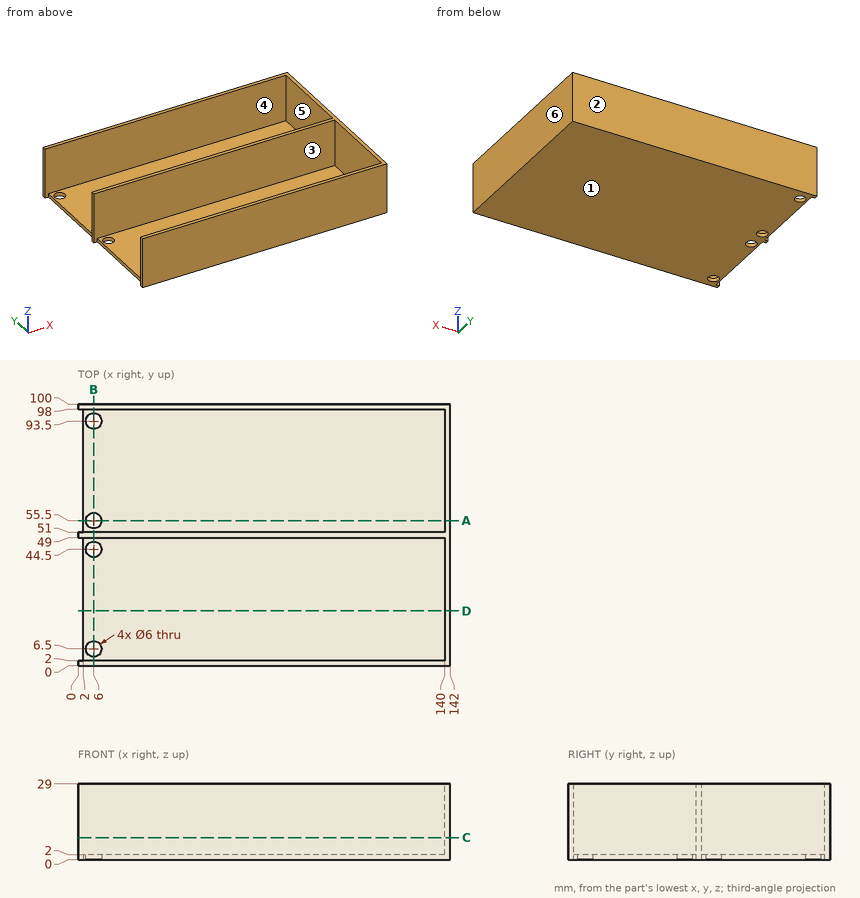
Input: dimensioned drawing with shaded views. Units: mm. Origin: part minimum x, y, z. A direction names the side the tool comes from. Coordinates: 2 decimals unless noted, no trailing zeros. Write each loop counter-clockwise with the first axis right and the second up, starting at its lowest first coordinate (ties: lowest second). Pieces come first, ordered by that corner, then holes. Notation, with made-up numbers: (27, 41) -> (80, 41) arc R37 cw to (80, 79) -> close; hole circle Ø5 at (64.5, 28). An arc over 180 degrees is marked (long way). Return JSON: item names as keys, results as strings. Group by question number.
1) Section query B-B, the plane x = 6. Return loops of the section in (y, z).
2) Section query D-D, the plane y = 21. Return loops of the section in (x, z), plus the area to 3 significant figures.
3) Section query C-C, the plane z = 8.5. Return loops of the section in (x, y), plus the area to 3 significant figures.
4) Contact query for flat-ended pins moving along their axis: P1, Ø14.5, axis at x = 97.5, z = 20, coming from the -Y side; P2, Ø8, axis at x = 6, y = 6.5, coming from the +Z side; P3, Ø0.6, axis at y = 72, z = 1, coming from the -X side; P4, Ø1, axis at y = 81.5, z = 16.5, coming from the -X side. Output: stop coordinate, or through.
5) Set-up query: the marked faces 5 and 6. Return all of +Z, -Z, +X, -X, +Y, -Y with unobstructed straight access to the full face (end or side cutting, diameter ignored); none if empty.
6) Section query A-A, the plane y = 55.5. Return loops of the section in (x, z), plus the area to 3 significant figures.
7) Ray query, line 1 along Y through (x, z) = (38.5, 7.75); line 2 along Y through (x, z) = (6, 0.6); line 3 along X through (y, z) = (12.5, 18). Return the intervals inside material, ascending.
8) Mould query, pull axis Y, two halves, no side actions, for the marked faces 1, 2, 3 and 4. Classes: +Y half, -Y half, draft (parallel to the pull), parting line (faces both ways), or undercut.
From the geometry:
{
 "1": {"outline": "(0, 0) -> (3.5, 0) -> (3.5, 2) -> (2, 2) -> (2, 29) -> (0, 29) -> close; (9.5, 0) -> (41.5, 0) -> (41.5, 2) -> (9.5, 2) -> close; (47.5, 0) -> (52.5, 0) -> (52.5, 2) -> (51, 2) -> (51, 29) -> (49, 29) -> (49, 2) -> (47.5, 2) -> close; (58.5, 0) -> (90.5, 0) -> (90.5, 2) -> (58.5, 2) -> close; (96.5, 0) -> (100, 0) -> (100, 29) -> (98, 29) -> (98, 2) -> (96.5, 2) -> close"},
 "2": {"outline": "(2, 0) -> (142, 0) -> (142, 29) -> (140, 29) -> (140, 2) -> (2, 2) -> close", "area": "334 mm²"},
 "3": {"outline": "(0, 0) -> (142, 0) -> (142, 100) -> (0, 100) -> (0, 98) -> (140, 98) -> (140, 51) -> (0, 51) -> (0, 49) -> (140, 49) -> (140, 2) -> (0, 2) -> close", "area": "1,040 mm²"},
 "4": {"P1": "y = 0", "P2": "z = 2", "P3": "x = 2", "P4": "x = 140"},
 "5": {"face 5": "+Z, -X", "face 6": "+Z, -Z, +X, +Y, -Y"},
 "6": {"outline": "(2, 0) -> (3, 0) -> (3, 2) -> (2, 2) -> close; (9, 0) -> (142, 0) -> (142, 29) -> (140, 29) -> (140, 2) -> (9, 2) -> close", "area": "322 mm²"},
 "7": {"line 1": "0 to 2, 49 to 51, 98 to 100", "line 2": "0 to 3.5, 9.5 to 41.5, 47.5 to 52.5, 58.5 to 90.5, 96.5 to 100", "line 3": "140 to 142"},
 "8": {"face 1": "draft", "face 2": "+Y half", "face 3": "undercut", "face 4": "undercut"}
}
